Geometry check sheet. Reference: the model listing, model coordinates, mm. Face numbers are marked on the shaded views. Coordinates: 2 decimals unless noted, no trailing zeros. Loops run counter-clockwise (first coordinate to the right, second up) from the corner with the lowest first, then second, coordinate; pieces in that order, holes last. Notation, with made-up numbers: M 40,72 L 73,72 A20 cw 73,90 Z; hole C 35.25,60.5 d2. An arc over 180 degrees is marked long. One line per question, with ' | ' between items. Start each with the question number.
from build123d import *

# Parameters (mm, degrees)
HOLE001_D           = 10
HOLE001_CBORE_D     = 14.5
HOLE001_CBORE_DEPTH = 10.3
FILLET001_R         = 0.5


with BuildPart() as part:
    # Sketch011 → Revolution003 (revolve)
    with BuildSketch(Plane.XZ):
        with BuildLine():
            Line((0, 0), (-11.5, 0))
            Line((-11.5, 0), (-11.5, 9.2))
            ThreePointArc((-11.5, 9.2), (-6.347978, 8.936721), (-1.3, 10))
            Line((0, 10), (-1.3, 10))
            Line((0, 0), (0, 10))
        make_face()
    revolve(axis=Axis((0, 0, 0), (1, 0, 0)))

    # Hole001 (through all)
    with Locations(Plane(origin=(-11.5, 0, 0), x_dir=(0, 0, -1), z_dir=(-1, 0, 0))):
        with Locations((0, 0)):
            CounterBoreHole(HOLE001_D / 2, HOLE001_CBORE_D / 2, HOLE001_CBORE_DEPTH)

    # Fillet001
    fillet001_edges = [part.edges().sort_by_distance(p)[0] for p in [
        (-11.5, 0, -9.2),
    ]]
    fillet(fillet001_edges, radius=FILLET001_R)


solid = part.part
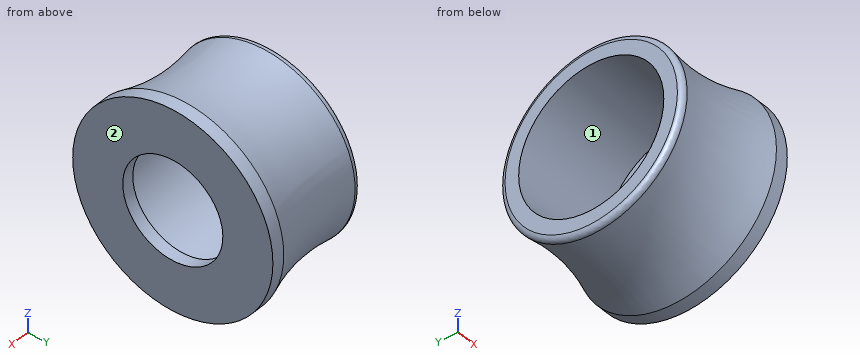
1. Sectioned sample at B-B (x = -9.25). Record the cut outline in (y, z), and give its area (3 significant figures).
2. Sectioned sample at A-A (x = -8). Record the cut outline in (y, z), and give its area (3 significant figures).
3. Depth check by flat-ended pin: pin 1 Ø12 at (y, z) = (5, 5) entering from -X; pin 2 Ø4 at (x, y) = (-2, 5.5) entering from +Z; pin 3 Ø1.5 at (x, z) = (-8.5, 0) entering from +Y; pin 4 Ø1 at (y, z) = (1.5, -3.5) entering from +X. Enter the tip coordinate at first touch or a pass-through.
4. Thickness scan on line 1 (Y direction, x = -0.25, z = 0); line 2 (X direction, y = -2.75, z = -5.5); line 3 (Z direction, x = -5.5, y = 4). Record the ranges inside material, lowest first.
5. Draft check along Y on the marked faces 1 and 2. Enter one of: +Y half, -Y half, draft (parallel to the pull), parting line (faces both ways), or undercut.
Result:
1) outline: C 0,0 d17.84; hole C 0,0 d14.5 | area: 84.9 mm2
2) outline: C 0,0 d17.75; hole C 0,0 d14.5 | area: 82.4 mm2
3) pin 1: stops at x = -11.5 | pin 2: stops at z = 9.32 | pin 3: stops at y = 8.92 | pin 4: passes through
4) line 1: y = -10 to -5, 5 to 10 | line 2: x = -1.2 to 0 | line 3: z = -8.09 to -6.05, 6.05 to 8.09
5) face 1: undercut | face 2: draft
